Model file for the job. Use its own axes, mm. Face numbers are marked on the shaded views. A direction names the side the tool comes from. Round coordinates to 2 decimals unless told otherwise and drop trailing zeros. Write each loop counter-clockwise with the first axis right and the second up, starting at its lowest first coordinate (ties: lowest second). Pieces come first, ordered by that corner, then holes. Notation, with made-up numbers: (41, -27.5) - (100, -27.5) arc R12 cw to (100, -16.5) - close; hole circle Ø3 at (0, 60.25). An arc over 180 degrees is marked (long way). One line per item, written item: value.
from build123d import *

# Parameters (mm, degrees)
ESQUISSE1_R                  = 105
BOSS_EXTRU_1_DEPTH           = 38
ENL_V_MAT_EXTRU_1_DEPTH      = 154.277526076
ENL_V_MAT_EXTRU_1_DEPTH_BACK = 154.277526076
ENL_V_MAT_EXTRU_2_DEPTH      = 154.277526076
ENL_V_MAT_EXTRU_2_DEPTH_BACK = 154.277526076
ESQUISSE3_R                  = 10
ESQUISSE4_R                  = 14
ENL_V_MAT_EXTRU_3_DEPTH      = 8.5
ENL_V_START                  = -29.5
ESQUISSE4_2_R                = 14
ENL_V_MAT_EXTRU_4_DEPTH      = 8.5
CONG_1_R                     = 4
ESQUISSE5_R                  = 105
ENL_V_MAT_EXTRU_5_DEPTH      = 19


with BuildPart() as part:
    # Esquisse1 → Boss.-Extru.1 (new body)
    with BuildSketch(Plane.XY):
        Circle(ESQUISSE1_R)
    extrude(amount=BOSS_EXTRU_1_DEPTH)

    # Esquisse2 → Enlèv. mat.-Extru.1 (cut, two sides: drawn at the far end of the back side and taken through both)
    with BuildSketch(Plane.XY.offset(38).offset(-ENL_V_MAT_EXTRU_1_DEPTH_BACK)):
        with BuildLine():
            Line((5.377682111, 24.414760599), (38.563838113, 70.091585729))
            ThreePointArc((38.563838113, 70.091585729), (0, 80), (-38.563838113, 70.091585729))
            Line((-38.563838113, 70.091585729), (-5.377682111, 24.414760599))
            ThreePointArc((-5.377682111, 24.414760599), (0, 25), (5.377682111, 24.414760599))
        make_face()
        with BuildLine():
            Line((24.881612324, 2.430096324), (78.57794069, -15.016898377))
            ThreePointArc((78.57794069, -15.016898377), (76.084521304, 24.72135955), (54.744178, 58.335880683))
            Line((54.744178, 58.335880683), (21.558021999, 12.659055553))
            ThreePointArc((21.558021999, 12.659055553), (23.776412907, 7.725424859), (24.881612324, 2.430096324))
        make_face()
        with BuildLine():
            Line((10, -22.912878475), (10, -79.372539332))
            ThreePointArc((10, -79.372539332), (47.022820183, -64.72135955), (72.397600803, -34.038028703))
            Line((72.397600803, -34.038028703), (18.701272437, -16.591034002))
            ThreePointArc((18.701272437, -16.591034002), (14.694631307, -20.225424859), (10, -22.912878475))
        make_face()
        with BuildLine():
            Line((-18.701272437, -16.591034002), (-72.397600803, -34.038028703))
            ThreePointArc((-72.397600803, -34.038028703), (-47.022820183, -64.72135955), (-10, -79.372539332))
            Line((-10, -79.372539332), (-10, -22.912878475))
            ThreePointArc((-10, -22.912878475), (-14.694631307, -20.225424859), (-18.701272437, -16.591034002))
        make_face()
        with BuildLine():
            Line((-21.558021999, 12.659055553), (-54.744178, 58.335880683))
            ThreePointArc((-54.744178, 58.335880683), (-76.084521304, 24.72135955), (-78.57794069, -15.016898377))
            Line((-78.57794069, -15.016898377), (-24.881612324, 2.430096324))
            ThreePointArc((-24.881612324, 2.430096324), (-23.776412907, 7.725424859), (-21.558021999, 12.659055553))
        make_face()
    extrude(amount=ENL_V_MAT_EXTRU_1_DEPTH + ENL_V_MAT_EXTRU_1_DEPTH_BACK, mode=Mode.SUBTRACT)

    # Esquisse3 → Enlèv. mat.-Extru.2 (cut, two sides: drawn at the far end of the back side and taken through both)
    with BuildSketch(Plane.XY.offset(38).offset(-ENL_V_MAT_EXTRU_2_DEPTH_BACK)):
        Circle(ESQUISSE3_R)
    extrude(amount=ENL_V_MAT_EXTRU_2_DEPTH + ENL_V_MAT_EXTRU_2_DEPTH_BACK, mode=Mode.SUBTRACT)

    # Esquisse4 → Enlèv. mat.-Extru.3 (cut)
    with BuildSketch(Plane.XY.offset(38)):
        Circle(ESQUISSE4_R)
    extrude(amount=-ENL_V_MAT_EXTRU_3_DEPTH, mode=Mode.SUBTRACT)

    # Esquisse4<2> → Enlèv. mat.-Extru.4 (cut)
    with BuildSketch(Plane.XY.offset(38).offset(ENL_V_START)):
        Circle(ESQUISSE4_2_R)
    extrude(amount=-ENL_V_MAT_EXTRU_4_DEPTH, mode=Mode.SUBTRACT)

    # Congé1
    cong_1_edges = [part.edges().sort_by_distance(p)[0] for p in [
        (-78.57794069, -15.016898377, 19),
        (-54.744178, 58.335880683, 19),
        (-21.558021999, 12.659055553, 19),
        (-24.881612324, 2.430096324, 19),
        (-10, -79.372539332, 19),
        (-72.397600803, -34.038028703, 19),
        (-18.701272437, -16.591034002, 19),
        (-10, -22.912878475, 19),
        (72.397600803, -34.038028703, 19),
        (10, -79.372539332, 19),
        (10, -22.912878475, 19),
        (18.701272437, -16.591034002, 19),
        (54.744178, 58.335880683, 19),
        (78.57794069, -15.016898377, 19),
        (24.881612324, 2.430096324, 19),
        (21.558021999, 12.659055553, 19),
        (-38.563838113, 70.091585729, 19),
        (38.563838113, 70.091585729, 19),
        (5.377682111, 24.414760599, 19),
        (-5.377682111, 24.414760599, 19),
    ]]
    fillet(cong_1_edges, radius=CONG_1_R)

    # Esquisse5 → Enlèv. mat.-Extru.5 (cut)
    with BuildSketch(Plane(origin=(0, 0, 0), x_dir=(-1, 0, 0), z_dir=(0, 0, -1))):
        Circle(ESQUISSE5_R)
    extrude(amount=-ENL_V_MAT_EXTRU_5_DEPTH, mode=Mode.SUBTRACT)


solid = part.part
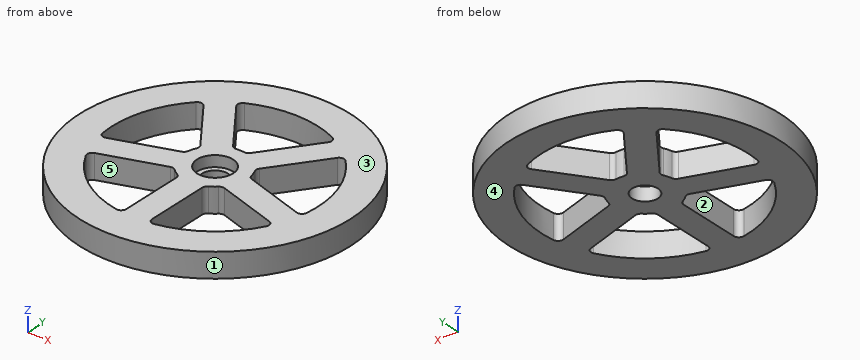
1. Band-saw the part on D-D on x = 82.5. Write the cut outline in (y, z).
Report:
outline: (-64.95, 19) - (64.95, 19) - (64.95, 38) - (-64.95, 38) - close
2. Band-saw the part on A-A on x = 0. Write the cut outline in (y, z), plus the area to 3 significant figures.
Report:
outline: (-105, 19) - (-10, 19) - (-10, 29.5) - (-14, 29.5) - (-14, 38) - (-105, 38) - close; (10, 19) - (25, 19) - (25, 38) - (14, 38) - (14, 29.5) - (10, 29.5) - close; (80, 19) - (105, 19) - (105, 38) - (80, 38) - close
area: 2,500 mm²
3. Band-saw the part on C-C on z = 23. State how many separate pieces and enclosed holes the cut face has, plus the area to 3 significant figures.
Report:
separate pieces: 1
enclosed holes: 6
area: 21,800 mm²
4. Drop flat-ended pins along their axis: pin 1 (3 mm diameter, centred on x = 17.5, z = 21, fed in from -Y); pin 2 (1.5 mm diameter, centred on x = -55, z = 26.5, fed in from -Y); pin 3 (1.5 mm diameter, centred on x = 24, z = 29.5, fed in from -Y). Give the stop position or say it passes through.
Report:
pin 1: y = -103.77
pin 2: y = -89.9
pin 3: y = -102.39
5. Tool access for the marked faces 4 and 5: list every direction of +Z, -Z, +X, -X, +Y, -Y with a clear straight run to the whole face (end or side of a thin tool).
Report:
face 4: -Z, +X, -X, +Y, -Y
face 5: +Z, -Z
6. Mould opens along Y. For the marked faces 1, 2 and 3 say: released by +Y, released by -Y, zero draft, split by the parting line, or undercut.
Report:
face 1: split by the parting line
face 2: undercut
face 3: zero draft
7. Band-saw the part on B-B on y = -67.5. Write the cut outline in (x, z).
Report:
outline: (-80.43, 19) - (-42.94, 19) - (-42.94, 38) - (-80.43, 38) - close; (-10, 19) - (10, 19) - (10, 38) - (-10, 38) - close; (42.94, 19) - (80.43, 19) - (80.43, 38) - (42.94, 38) - close
8. Wall check: probe 1 along Y at (x, z) = (0, 33); probe 2 along Y at (x, z) = (0, 26); probe 3 along X at (y, z) = (-67, 22). Give the ranges that are in metal, low to high. Write a range as [from, to].
Report:
probe 1: [-105, -14], [14, 25], [80, 105]
probe 2: [-105, -10], [10, 25], [80, 105]
probe 3: [-80.85, -43.71], [-10, 10], [43.71, 80.85]
